Can you work these out from the model? Positions are in its coordinate system, mm. Face numbers are marked on the shaded views. A direction names the side the tool comes from. Round coordinates to 2 decimals unless told otherwise and drop trailing zeros. Loops run counter-clockwise (first coordinate to the right, second up) from the corner with the lowest first, then second, coordinate; pieces in that order, holes last. Notation, with made-up numbers: (0.25, -12.5) -> (21.25, -12.5) arc R15 ccw to (21.25, 10.5) -> close; hole circle Ø6 at (-5.5, 47.25). An arc over 180 degrees is marked (long way). Use a Markdown table: item, result.
from build123d import *

# Parameters (mm, degrees)
SKETCH1_W           = 100
SKETCH1_H           = 78
BOSS_EXTRUDE1_DEPTH = 30
SKETCH3_W           = 82
SKETCH3_H           = 54
CUT_EXTRUDE1_DEPTH  = 3
SHELL1_T            = -3
FILLET1_R           = 5
FILLET2_R           = 5


with BuildPart() as part:
    # Sketch1 → Boss-Extrude1 (new body)
    with BuildSketch(Plane.XY):
        with Locations((8.119223597, 15.253918495)):
            Rectangle(SKETCH1_W, SKETCH1_H)
    extrude(amount=-BOSS_EXTRUDE1_DEPTH)

    # Sketch3 → Cut-Extrude1 (cut)
    with BuildSketch(Plane.XY):
        with Locations((8.119223597, 15.253918495)):
            Rectangle(SKETCH3_W, SKETCH3_H)
    extrude(amount=-CUT_EXTRUDE1_DEPTH, mode=Mode.SUBTRACT)

    # Shell1
    shell1_openings = [part.faces().sort_by_distance(p)[0] for p in [
        (8.119223597, 15.253918495, -30),
    ]]
    offset(amount=SHELL1_T, openings=shell1_openings, kind=Kind.INTERSECTION)

    # Fillet1
    fillet1_edges = [part.edges().sort_by_distance(p)[0] for p in [
        (8.119223597, -23.746081505, 0),
        (-41.880776403, 15.253918495, 0),
        (8.119223597, 54.253918495, 0),
        (58.119223597, 15.253918495, 0),
        (58.119223597, -23.746081505, -15),
        (-41.880776403, -23.746081505, -15),
        (-41.880776403, 54.253918495, -15),
        (58.119223597, 54.253918495, -15),
    ]]
    fillet(fillet1_edges, radius=FILLET1_R)

    # Fillet2
    # the kernel refuses this fillet: 5 mm, written as the material it adds along each edge
    with BuildSketch(Plane(origin=(55.119223597, -20.746081505, -3), x_dir=(0, 0, -1), z_dir=(0, 1, 0))) as fillet2_piece_1:
        with BuildLine():
            CenterArc((FILLET2_R, FILLET2_R), FILLET2_R, 180, 90)
            Line((0, FILLET2_R), (0, 0))
            Line((0, 0), (FILLET2_R, 0))
        make_face()
    extrude(amount=72)
    with BuildSketch(Plane(origin=(-38.880776403, 51.253918495, -3), x_dir=(0, 0, -1), z_dir=(1, 0, 0))) as fillet2_piece_2:
        with BuildLine():
            CenterArc((FILLET2_R, -FILLET2_R), FILLET2_R, 90, 90)
            Line((0, -FILLET2_R), (0, 0))
            Line((0, 0), (FILLET2_R, 0))
        make_face()
    extrude(amount=94)


solid = part.part
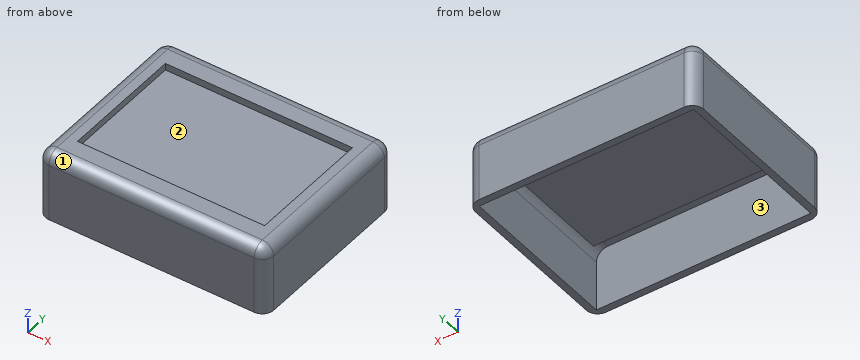
1. I want a section at D-D (y = -13.5). Please give me the cut outline in (x, z).
Answer sheet:
| item | result |
|---|---|
| outline | (-41.88, -30) -> (-38.88, -30) -> (-38.88, -3) -> (-35.88, -3) -> (-35.88, -6) -> (52.12, -6) -> (52.12, -3.42) arc R5 cw to (55.12, -8) -> (55.12, -30) -> (58.12, -30) -> (58.12, -5) arc R5 ccw to (53.12, 0) -> (-36.88, 0) arc R5 ccw to (-41.88, -5) -> close |
2. I want a section at A-A (y = 26). Please give me the cut outline in (x, z).
Answer sheet:
| item | result |
|---|---|
| outline | (-41.88, -30) -> (-38.88, -30) -> (-38.88, -3) -> (-35.88, -3) -> (-35.88, -6) -> (52.12, -6) -> (52.12, -3.42) arc R5 cw to (55.12, -8) -> (55.12, -30) -> (58.12, -30) -> (58.12, -5) arc R5 ccw to (53.12, 0) -> (49.12, 0) -> (49.12, -3) -> (-32.88, -3) -> (-32.88, 0) -> (-36.88, 0) arc R5 ccw to (-41.88, -5) -> close |
3. I need wall thicknesses on line 1 (Y direction, x = 39.5, z = -14.25); line 2 (X direction, y = 32, z = -17.5); line 3 (Y direction, x = -22.5, z = -5.25). Which ranges of each line are inside material? Lowest first, please.
Answer sheet:
| item | result |
|---|---|
| line 1 | y = -23.75 to -20.75, 51.25 to 54.25 |
| line 2 | x = -41.88 to -38.88, 55.12 to 58.12 |
| line 3 | y = -23.75 to -20.75, -14.75 to 45.25, 50.43 to 54.25 |
4. Will these pins go through, and if not, where does the flat tip stop? pin 1 Ø3.5 at (x, z) = (26, -1.5) entering from -Y; pin 2 Ø1 at (x, y) = (-29, -8.5) entering from +Z; pin 3 Ø3 at (x, y) = (-26, 13.5) entering from -Z.
Answer sheet:
| item | result |
|---|---|
| pin 1 | stops at y = -23.43 |
| pin 2 | stops at z = -3 |
| pin 3 | stops at z = -6 |
5. Which directions (+Z, -Z, +X, -X, +Y, -Y) give clear straight access to the entire face, cutting with the end or side of a thin tool? Please do the marked faces 1, 2 and 3.
Answer sheet:
| item | result |
|---|---|
| face 1 | +Z, +X, -X, -Y |
| face 2 | +Z |
| face 3 | -Z |
6. I want a section at B-B (z = -16.75). Please give me the cut outline in (x, y).
Answer sheet:
| item | result |
|---|---|
| outline | (-41.88, -18.75) arc R5 ccw to (-36.88, -23.75) -> (53.12, -23.75) arc R5 ccw to (58.12, -18.75) -> (58.12, 49.25) arc R5 ccw to (53.12, 54.25) -> (-36.88, 54.25) arc R5 ccw to (-41.88, 49.25) -> close; hole (-38.88, -20.75) -> (55.12, -20.75) -> (55.12, 51.25) -> (-38.88, 51.25) -> close |
7. I want a section at C-C (x = 33). Please give me the cut outline in (y, z).
Answer sheet:
| item | result |
|---|---|
| outline | (-23.75, -30) -> (-20.75, -30) -> (-20.75, -3) -> (-14.75, -3) -> (-14.75, -6) -> (45.25, -6) -> (45.25, -3) -> (46.25, -3) arc R5 cw to (51.25, -8) -> (51.25, -30) -> (54.25, -30) -> (54.25, -5) arc R5 ccw to (49.25, 0) -> (42.25, 0) -> (42.25, -3) -> (-11.75, -3) -> (-11.75, 0) -> (-18.75, 0) arc R5 ccw to (-23.75, -5) -> close |
